Can you work these out from the model? Positions are in its coordinate system, mm. Face numbers are marked on the shaded views. A direction names the side the tool comes from. Give positions to 0.01 mm unless a question says otherwise; leave off trailing zeros. Order: outer loops, then holes, each group sorted by start corner. A loop starts at its lowest first (then second) coordinate and runs counter-clockwise, first axis right, second up. Notation, with made-up numbers: (9, 33) -> (24, 33) arc R20 cw to (24, 65) -> close; hole circle Ø11 at (68.5, 29). An arc over 180 degrees is marked (long way). Answer as a JSON object with one key per item and string values.
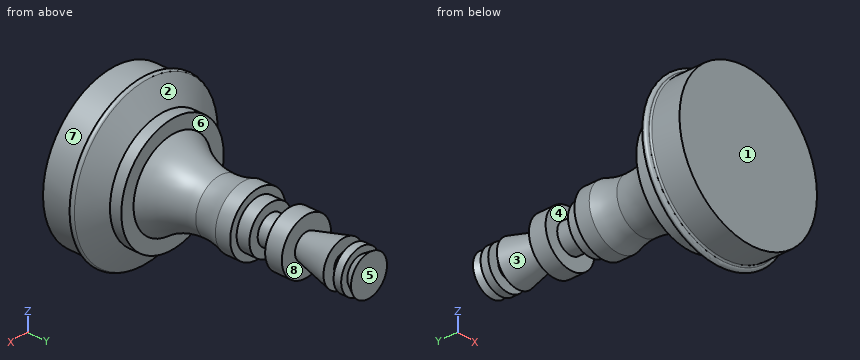
```python
from build123d import *

# Parameters (mm, degrees)
SCALE_1_SCALE = 1.5


with BuildPart() as part:
    # 草圖2 → 旋轉1 (revolve)
    with BuildSketch(Plane.XY, mode=Mode.PRIVATE) as revolve_1_sk:
        with BuildLine():
            Line((0, 0), (135.201465244, 0))
            Line((135.201465244, 0), (135.201465244, 48.846470305))
            ThreePointArc((135.201465244, 48.846470305), (135.933698291, 50.614237258), (137.701465244, 51.346470305))
            Line((137.701465244, 51.346470305), (138.117818628, 51.346470305))
            ThreePointArc((138.117818628, 51.346470305), (142.905095232, 54.903562575), (140.880857994, 60.513677218))
            Line((140.880857994, 60.513677218), (100.681841945, 87.167372643))
            Line((100.681841945, 87.167372643), (100.681841945, 107.133121487))
            Line((100.681841945, 107.133121487), (76.60549775, 107.133121487))
            ThreePointArc((76.60549775, 107.133121487), (54.387004145, 145.940882587), (46.656874484, 189.985733309))
            ThreePointArc((46.656874484, 189.985733309), (48.623022714, 211.196335783), (54.479774894, 231.676908287))
            Line((54.479774894, 231.676908287), (54.479774894, 257.848515079))
            Line((54.479774894, 257.848515079), (41.803489055, 257.848515079))
            Line((41.803489055, 257.848515079), (41.803489055, 280.427838471))
            Line((41.803489055, 280.427838471), (25.557390517, 280.427838471))
            Line((25.557390517, 280.427838471), (25.557390517, 314.091902385))
            Line((25.557390517, 314.091902385), (48.412071511, 314.091902385))
            Line((48.412071511, 314.091902385), (48.412071511, 343.442796825))
            Line((48.412071511, 343.442796825), (22.495215746, 343.442796825))
            Line((22.495215746, 343.442796825), (39.007295277, 408.518950092))
            Line((39.007295277, 408.518950092), (17.96096835, 408.518950092))
            Line((17.96096835, 408.518950092), (17.96096835, 425.053771457))
            Line((17.96096835, 425.053771457), (37.557793671, 425.053771457))
            Line((37.557793671, 425.053771457), (37.557793671, 438.526588864))
            Line((37.557793671, 438.526588864), (25.557390517, 438.526588864))
            Line((25.557390517, 438.526588864), (35.414390901, 453.836608646))
            Line((35.414390901, 453.836608646), (0, 453.836608646))
            Line((0, 453.836608646), (0, 0))
        make_face()
    revolve(revolve_1_sk.sketch.rotate(Axis((0, 453.836608646, 0), (0, -1, 0)), 180), axis=Axis((0, 453.836608646, 0), (0, -1, 0)))


with BuildPart() as part_1:
    # 縮放比例1: scaled about (0, 100.72058529, 0)
    add(part.part.scale(SCALE_1_SCALE).moved(Location((0, -50.360292645, 0))))


solid = part_1.part
```
1. Please list where these lines run through material, in increasing order: L1, parallel to Y at x = 65, z = 21; L2, parallel to Y at x = 116, z = -55.5; L3, parallel to Z at x = -135.5, y = -5.
Worked answers:
{"L1": "-50.36 to 336.41, 420.78 to 464.8", "L2": "-50.36 to 110.34", "L3": "-150.89 to 150.89"}
2. If we section it at A-A on y = 437: Please give me the cut outline in (x, z), then the cut area to 3 significant figures.
Worked answers:
{"outline": "circle Ø145.24 at (0, 0)", "area": "16,600 mm²"}
3. For the marked faces 5, 6, 7 and 8, which set-ups out of +Z, -Z, +X, -X, +Y, -Y let a thin tool reach every point of the face, with its end or its side?
Worked answers:
{"face 5": "+Z, -Z, +X, -X, +Y", "face 6": "+Y", "face 7": "-Y", "face 8": "none"}
4. Will these pins go through, and if not, where does the flat tip stop? pin 1 Ø2 at (x, y) = (-18.5, 321.5) entering from -Z; pin 2 Ø6 at (y, z) = (288, 8) entering from +X; pin 3 Ø12 at (y, z) = (260.5, -68) entering from +X.
Worked answers:
{"pin 1": "z = -79.82", "pin 2": "x = 79.09", "pin 3": "x = 36.63"}
5. If we mould it in two halves opening along Y, with no side actions, what happens to the marked faces 1, 2, 3 and 4? For each: +Y half, -Y half, draft (parallel to the pull), parting line (faces both ways), or undercut.
Worked answers:
{"face 1": "-Y half", "face 2": "+Y half", "face 3": "undercut", "face 4": "undercut"}
6. If we section it at B-B on y = 1: Please give me the cut outline in (x, z).
Worked answers:
{"outline": "circle Ø405.6 at (0, 0)"}
